For this review, take the finished solid that the model builds, in its own axes (mm). A direction names the side the tool comes from. Round coordinates to 2 decimals unless told otherwise and drop trailing zeros. Order: outer loops, then holes, each group sorted by start corner. A loop starts at its lowest first (then second) coordinate and runs counter-clockwise, first axis right, second up. Notation, with made-up numbers: M -25,53.25 L -5,53.25 A31 ccw -5,84.25 Z; hole C -9.5,76.5 d3. An arc over 180 degrees is marked long. Answer as a JSON object with one key per item and string values.
from build123d import *

# Parameters (mm, degrees)
SKETCH1_W           = 44
SKETCH1_H           = 21
SKETCH1_R           = 1.35
BOSS_EXTRUDE1_DEPTH = 1
SKETCH2_W           = 36
SKETCH2_H           = 19
BOSS_EXTRUDE2_DEPTH = 0.5
FILLET1_R           = 3
SKETCH3_W           = 6
SKETCH3_H           = 23
BOSS_EXTRUDE3_DEPTH = 7


with BuildPart() as part:
    # Sketch1 → Boss-Extrude1 (new body)
    with BuildSketch(Plane.XY):
        Rectangle(SKETCH1_W, SKETCH1_H)
        with Locations((-20, 8.25)):
            Circle(SKETCH1_R, mode=Mode.SUBTRACT)
        with Locations((-20, -8.25)):
            Circle(SKETCH1_R, mode=Mode.SUBTRACT)
    extrude(amount=BOSS_EXTRUDE1_DEPTH)

    # Sketch2 → Boss-Extrude2 (add)
    with BuildSketch(Plane.XY.offset(1)):
        with Locations((0.25, 0)):
            Rectangle(SKETCH2_W, SKETCH2_H)
    extrude(amount=BOSS_EXTRUDE2_DEPTH)

    # Fillet1
    fillet1_edges = [part.edges().sort_by_distance(p)[0] for p in [
        (18.25, 9.5, 1.25),
        (-17.75, 9.5, 1.25),
        (-17.75, -9.5, 1.25),
        (18.25, -9.5, 1.25),
    ]]
    fillet(fillet1_edges, radius=FILLET1_R)

    # Sketch3 → Boss-Extrude3 (add)
    with BuildSketch(Plane(origin=(0, 0, 0), x_dir=(-1, 0, 0), z_dir=(0, 0, -1))):
        with Locations((-21.5, 0)):
            Rectangle(SKETCH3_W, SKETCH3_H)
    extrude(amount=BOSS_EXTRUDE3_DEPTH)


solid = part.part
1) Machinability: for faces 1 (the cylindrical face through (17.39, 8.6, 1.25)), 2 (the cylindrical face through (-16.85, -8.64, 1.25)), 3 (the flat face through (22, -0.1, 0.5)), which of the approach directions +Z, -Z, +X, -X, +Y, -Y give a long, thin tool a straight path to every point of the face, cutting with its end or side? Answer none if there is none.
Geometry check:
{"face 1": "+Z, +X, +Y", "face 2": "+Z, -X, -Y", "face 3": "+Z, +X, +Y, -Y"}
2) Add section B-B on y = -8.25. State the section outline as (x, z) points, and give its area (3 significant figures).
Geometry check:
{"outline": "M -22,0 L -21.35,0 L -21.35,1 L -22,1 Z; M -18.65,0 L 18.5,0 L 18.5,-7 L 24.5,-7 L 24.5,0 L 22,0 L 22,1 L 17.69,1 L 17.69,1.5 L -17.19,1.5 L -17.19,1 L -18.65,1 Z", "area": "101 mm²"}
3) Add section C-C on y = 0.75. State the section outline as (x, z) points, and give its area (3 significant figures).
Geometry check:
{"outline": "M -22,0 L 18.5,0 L 18.5,-7 L 24.5,-7 L 24.5,0 L 22,0 L 22,1 L 18.25,1 L 18.25,1.5 L -17.75,1.5 L -17.75,1 L -22,1 Z", "area": "104 mm²"}
4) Add section A-A on x = -20. State the section outline as (y, z) points, and give its area (3 significant figures).
Geometry check:
{"outline": "M -10.5,0 L -9.6,0 L -9.6,1 L -10.5,1 Z; M -6.9,0 L 6.9,0 L 6.9,1 L -6.9,1 Z; M 9.6,0 L 10.5,0 L 10.5,1 L 9.6,1 Z", "area": "15.6 mm²"}
5) Add section D-D on x = -14. State the section outline as (y, z) points.
Geometry check:
{"outline": "M -10.5,0 L 10.5,0 L 10.5,1 L 9.5,1 L 9.5,1.5 L -9.5,1.5 L -9.5,1 L -10.5,1 Z"}
6) For L1, parallel to Y at x = -20, z = 0.4; L2, parallel to X at y = 0, z = -0.5; L3, parallel to Z at x = 12, y = 7, list the stretches that pass through material, from the lowest coordinate up.
Geometry check:
{"L1": "y = -10.5 to -9.6, -6.9 to 6.9, 9.6 to 10.5", "L2": "x = 18.5 to 24.5", "L3": "z = 0 to 1.5"}
7) Mouldability with a two-part tool opening along X and no side actions: class faces 4 (the cylindrical face through (-19.274, -7.112, 0.493)), 5 (the flat face through (-2, 0, 0)), 6 (the cylindrical face through (17.35, -8.64, 1.25)), 7 (the cylindrical face through (-16.85, 8.64, 1.25)) as +X half, -X half, draft (parallel to the pull), parting line (faces both ways), or undercut.
Geometry check:
{"face 4": "undercut", "face 5": "draft", "face 6": "+X half", "face 7": "-X half"}
8) Insertion check: P1, Ø3, axis at x = -17, z = -1, coming from the -Y side; P2, Ø3, axis at y = -1, z = -3.5, coming from the -X side; P3, Ø0.8, axis at y = -0.5, z = 0.5, coming from the +X side. Each pin has a flat end and moves straight along its axis. Give the tip position at first contact, or say it passes through.
Geometry check:
{"P1": "stops at y = -10.5", "P2": "stops at x = 18.5", "P3": "stops at x = 22"}
